Can you work these out from the model? Positions are in its coordinate system, mm. Face numbers are marked on the shaded views. Give positions to 0.01 mm unless a question says otherwise; leave off trailing zeros. Order: outer loops, then holes, each group sorted by start corner. A loop starts at its lowest first (then second) coordinate and runs counter-clockwise, first axis right, second up. Notation, with made-up numbers: (69, 66.5) - (103, 66.5) arc R28 ccw to (103, 99.5) - close; hole circle Ø9 at (31.5, -15). An arc over 180 degrees is marked (long way). One line per question, with ' | ' between items.
```python
from build123d import *


with BuildPart() as part:
    # Sketch2 → Revolve1 (revolve)
    with BuildSketch(Plane(origin=(0, 0, 0), x_dir=(1, 0, 0), z_dir=(0, 1, 0))):
        with BuildLine():
            Line((0, 0), (0, 8.001))
            ThreePointArc((0, 8.001), (-0.446369265, 9.078630735), (-1.524, 9.525))
            Line((-1.524, 9.525), (-7.9248, 9.525))
            Line((-7.9248, 9.525), (-7.9248, 11.1125))
            Line((-7.9248, 11.1125), (-9.525, 11.1125))
            Line((-9.525, 11.1125), (-9.525, 12.7))
            Line((-9.525, 12.7), (1.651, 12.7))
            ThreePointArc((1.651, 12.7), (2.728630735, 12.253630735), (3.175, 11.176))
            Line((3.175, 11.176), (3.175, 0))
            Line((3.175, 0), (0, 0))
        make_face()
    revolve(axis=Axis((3.175, 0, 0), (-1, 0, 0)))


solid = part.part
```
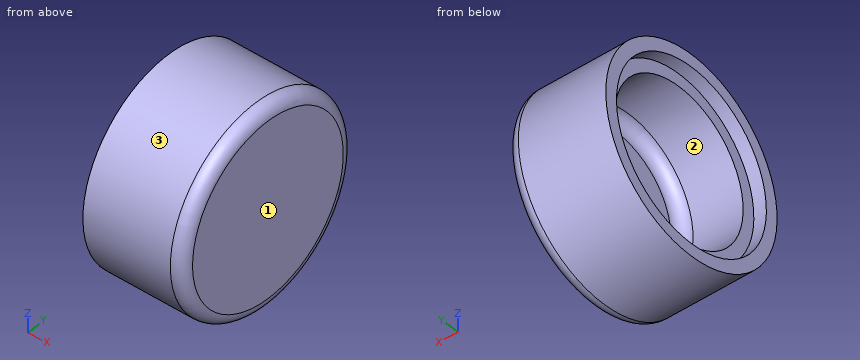
(1) If I drill on line 1 (Z direction, x = -6.25, y = 0) (3 decimals); line 2 (Z direction, x = -8.4, y = 0), over which ranges is the centre line in solid material (lowest first)?
Answer below:
line 1: -12.7 to -9.525, 9.525 to 12.7 | line 2: -12.7 to -11.11, 11.11 to 12.7
(2) Imagine slicing it at B-B (x = -8.25). List the corners of the cut face in (y, z) for me (1 decimal), and give its area (3 significant figures).
Answer below:
outline: circle Ø25.4 at (0, 0); hole circle Ø22.2 at (0, 0) | area: 119 mm^2
(3) Will these pins go through, and if not, where does the flat tip stop? pin 1 (1 mm diameter, centred on x = -2.5, z = 1.5, fed in from -Y); pin 2 (5 mm diameter, centred on x = 1, y = -6.5, fed in from -Z); pin 3 (6 mm diameter, centred on x = -6, y = -8, fed in from +Z).
Answer below:
pin 1: y = -12.66 | pin 2: z = -12.05 | pin 3: z = 11.67
(4) Imagine slicing it at A-A (z = 0). List the corners of the cut face in (x, y) for me (1 decimal).
Answer below:
outline: (-9.5, -12.7) - (1.7, -12.7) arc R1.5 ccw to (3.2, -11.2) - (3.2, 11.2) arc R1.5 ccw to (1.7, 12.7) - (-9.5, 12.7) - (-9.5, 11.1) - (-7.9, 11.1) - (-7.9, 9.5) - (-1.5, 9.5) arc R1.5 cw to (0, 8) - (0, -8) arc R1.5 cw to (-1.5, -9.5) - (-7.9, -9.5) - (-7.9, -11.1) - (-9.5, -11.1) - close
(5) If we mould it in two halves opening along Y, with no side actions, what happens to the marked faces 1, 2 and 3? For each: released by +Y, released by -Y, zero draft, split by the parting line, or undercut.
Answer below:
face 1: zero draft | face 2: undercut | face 3: split by the parting line
(6) Imagine slicing it at D-D (x = 0.5). List the corners of the cut face in (y, z) for me, and give its area (3 significant figures).
Answer below:
outline: circle Ø25.4 at (0, 0) | area: 507 mm^2
